For this review, take the finished solid that the model builds, in its own axes (mm). Round coordinates to 2 decimals unless told otherwise and drop trailing zeros. Write each loop counter-clockwise with the first axis right and the second up, starting at its lowest first coordinate (ties: lowest second). Pieces come first, ordered by that corner, then holes. Notation, with made-up numbers: M 29,38 L 50,38 A19 ccw 50,64 Z; hole C -22.75,22 d9. An arc over 180 degrees is marked long. Answer in a Markdown table with one row per item.
```python
from build123d import *

# Parameters (mm, degrees)
BOSS_EXTRUDE1_DEPTH = 3.175
SKETCH2_W           = 15
SKETCH2_H           = 3.175
CUT_EXTRUDE1_DEPTH  = 10
SKETCH3_W           = 50
SKETCH3_H           = 3.175
CUT_EXTRUDE2_DEPTH  = 10
SKETCH4_W           = 3.175
SKETCH4_H           = 10
CUT_EXTRUDE3_DEPTH  = 10


with BuildPart() as part:
    # Sketch1 → Boss-Extrude1 (new body)
    with BuildSketch(Plane.XY):
        Polygon((3.175, 0), (3.175, 55), (0, 55), (0, 135), (3.175, 135), (3.175, 205), (0, 205), (0, 235), (100, 235), (100, 220), (96.825, 220), (96.825, 150), (100, 150), (100, 110), (50, 110), (35, 110), (35, 106.825), (50, 106.825), (50, 86.825), (46.825, 86.825), (46.825, 36.825), (50, 36.825), (50, 20), (100, 20), (100, 0), align=None)
    extrude(amount=-BOSS_EXTRUDE1_DEPTH)

    # Sketch2 → Cut-Extrude1 (cut)
    with BuildSketch(Plane.XY):
        with Locations((72.5, 18.4125)):
            Rectangle(SKETCH2_W, SKETCH2_H)
    extrude(amount=-CUT_EXTRUDE1_DEPTH, mode=Mode.SUBTRACT)

    # Sketch3 → Cut-Extrude2 (cut)
    with BuildSketch(Plane.XY):
        with Locations((50, 233.4125)):
            Rectangle(SKETCH3_W, SKETCH3_H)
    extrude(amount=-CUT_EXTRUDE2_DEPTH, mode=Mode.SUBTRACT)

    # Sketch4 → Cut-Extrude3 (cut)
    with BuildSketch(Plane.XY):
        with Locations((98.4125, 10)):
            Rectangle(SKETCH4_W, SKETCH4_H)
    extrude(amount=-CUT_EXTRUDE3_DEPTH, mode=Mode.SUBTRACT)


solid = part.part
```
Q1. Insertion check: P1, Ø1.6, axis at x = 74, z = -2.5, coming from the +Y side (3 decimals); P2, Ø1.6, axis at y = 39, z = -1, coming from the -X side (3 decimals); P3, Ø1, axis at y = 57, z = -1.5, coming from the +X side (3 decimals). Each pin has a flat end and moves straight along its axis. Give the tip position at first contact, or say it passes through.
Found:
| item | result |
|---|---|
| P1 | y = 231.825 |
| P2 | x = 3.175 |
| P3 | x = 46.825 |
Q2. Take a section at C-C (y = 27.5). State the section outline as (x, z) points (3 decimals).
Found:
| item | result |
|---|---|
| outline | M 3.175,-3.175 L 50,-3.175 L 50,0 L 3.175,0 Z |
Q3. Take a section at D-D (y = 170.5). State the section outline as (x, z) points (3 decimals).
Found:
| item | result |
|---|---|
| outline | M 3.175,-3.175 L 96.825,-3.175 L 96.825,0 L 3.175,0 Z |
Q4. Take a section at A-A (x = 71.5). State the section outline as (y, z) points (3 decimals), then the cut area to 3 significant figures.
Found:
| item | result |
|---|---|
| outline | M 0,-3.175 L 16.825,-3.175 L 16.825,0 L 0,0 Z; M 110,-3.175 L 231.825,-3.175 L 231.825,0 L 110,0 Z |
| area | 440 mm² |
Q5. Take a section at B-B (x = 53.5). State the section outline as (y, z) points (3 decimals), then the cut area to 3 significant figures.
Found:
| item | result |
|---|---|
| outline | M 0,-3.175 L 20,-3.175 L 20,0 L 0,0 Z; M 110,-3.175 L 231.825,-3.175 L 231.825,0 L 110,0 Z |
| area | 450 mm² |
Q6. For probe 1 along Y at (x, z) = (48, -2) (3 decimals); probe 2 along Y at (x, z) = (62, -2.1) (3 decimals); probe 3 along Y at (x, z) = (84.5, -0.2), list the stretches that pass through material, from the lowest coordinate up.
Found:
| item | result |
|---|---|
| probe 1 | 0 to 36.825, 86.825 to 106.825, 110 to 231.825 |
| probe 2 | 0 to 20, 110 to 231.825 |
| probe 3 | 0 to 20, 110 to 235 |
